```python
from build123d import *

# Parameters (mm, degrees)
F1_DEPTH = 35
F2_R     = 1.85
F3_DEPTH = 6.001


# Not quite as in the source:
# - a feature names something its author has since deleted; it is built from what else it names


with BuildPart() as f1:
    # F0 (on Front) → F1 (new body, symmetric)
    with BuildSketch(Plane.XZ):
        Polygon((-10.06, 8), (-10.06, 10), (10.06, 10), (10.06, 8), (12.5, 8), (12.5, 14), (-12.5, 14), (-12.5, 8), align=None)
    extrude(amount=F1_DEPTH, both=True)

    # F2 (on face) → F3 (cut, through all)
    with BuildSketch(Plane.XY.offset(14)):
        Circle(F2_R)
    extrude(amount=-F3_DEPTH, mode=Mode.SUBTRACT)


solid = f1.part
```
Can you work these out from the model? Positions are in its coordinate system, mm. A direction names the side the tool comes from. Coordinates: 2 decimals unless noted, no trailing zeros. Loops run counter-clockwise (first coordinate to the right, second up) from the corner with the lowest first, then second, coordinate; pieces in that order, holes last. Notation, with made-up numbers: (78, 72.25) - (115, 72.25) arc R17 cw to (115, 82.25) - close; hole circle Ø7 at (-19.75, 86). An arc over 180 degrees is marked (long way). Use a Markdown table: item, result.
Item 1: For faces 1 (the face through (10.06, 0, 9)), 2 (the face through (-11, 0, 8)), which set-ups out of +Z, -Z, +X, -X, +Y, -Y let a thin tool reach every point of the face, with its end or its side?
Numbers:
| item | result |
|---|---|
| face 1 | -Z, +Y, -Y |
| face 2 | -Z, +X, -X, +Y, -Y |
Item 2: We'd pull the mould along X, two halves only. Please class faces 3 (the face through (-12.5, 0, 11)), 4 (the face through (12.5, 0, 11)), 5 (the face through (-0.401, -1.806, 12.028)), 6 (the face through (3, 0, 14)): released by +X, released by -X, zero draft, split by the parting line, or undercut.
Numbers:
| item | result |
|---|---|
| face 3 | released by -X |
| face 4 | released by +X |
| face 5 | undercut |
| face 6 | zero draft |
Item 3: I want a section at B-B on x = 0. Please give me the cut outline in (y, z), and give its area (3 significant figures).
Numbers:
| item | result |
|---|---|
| outline | (-35, 10) - (-1.85, 10) - (-1.85, 14) - (-35, 14) - close; (1.85, 10) - (35, 10) - (35, 14) - (1.85, 14) - close |
| area | 265 mm2 |
Item 4: If I drill on probe 1 along Y at (x, z) = (0, 12.3); probe 2 along X at (y, z) = (-22, 9.9); probe 3 along Z at (x, y) = (1.25, 15.5), over which ranges is the centre line in solid material (lowest first)? Write a range as from..to.
Numbers:
| item | result |
|---|---|
| probe 1 | y = -35..-1.85, 1.85..35 |
| probe 2 | x = -12.5..-10.06, 10.06..12.5 |
| probe 3 | z = 10..14 |
Item 5: I want a section at A-A on y = 0. Please give me the cut outline in (x, z).
Numbers:
| item | result |
|---|---|
| outline | (-12.5, 8) - (-10.06, 8) - (-10.06, 10) - (-1.85, 10) - (-1.85, 14) - (-12.5, 14) - close; (1.85, 10) - (10.06, 10) - (10.06, 8) - (12.5, 8) - (12.5, 14) - (1.85, 14) - close |
Item 6: Will this pin go through, and if not, where does the flat tip stop? pin 1 (3 mm diameter, centred on x = 1.5, y = 17, fed in from -Z).
Numbers:
| item | result |
|---|---|
| pin 1 | stops at z = 10 |
Item 7: I want a section at D-D on x = 3.25. Please give me the cut outline in (y, z), and give its area (3 significant figures).
Numbers:
| item | result |
|---|---|
| outline | (-35, 10) - (35, 10) - (35, 14) - (-35, 14) - close |
| area | 280 mm2 |
Item 8: I want a section at C-C on y = 13. Please give me the cut outline in (x, z).
Numbers:
| item | result |
|---|---|
| outline | (-12.5, 8) - (-10.06, 8) - (-10.06, 10) - (10.06, 10) - (10.06, 8) - (12.5, 8) - (12.5, 14) - (-12.5, 14) - close |
